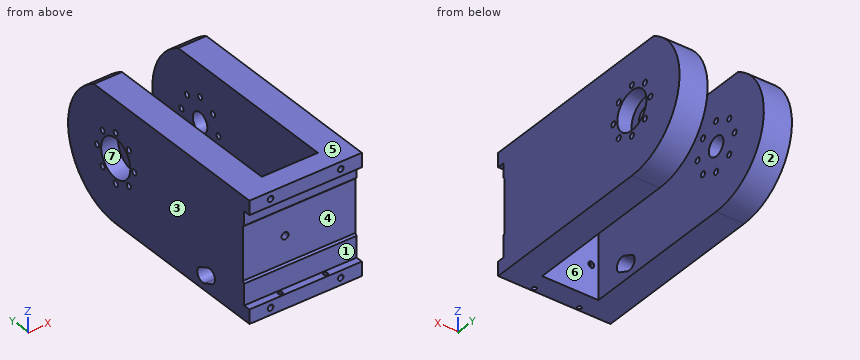
from build123d import *

# Parameters (mm, degrees)
BOSS_EXTRUDE1_DEPTH          = 101.6
CUT_EXTRUDE1_DEPTH           = 264.20443605
CUT_EXTRUDE1_DEPTH_BACK      = 264.20443605
SKETCH5_R                    = 17.4625
CUT_EXTRUDE4_DEPTH           = 15.24
CUT_EXTRUDE5_DEPTH           = 264.20443605
CUT_EXTRUDE5_DEPTH_BACK      = 264.20443605
SKETCH6_R                    = 8.73125
CUT_EXTRUDE6_START           = -12.85875
SKETCH7_R                    = 17.4625
CUT_EXTRUDE6_DEPTH           = 12.85875
F_1_4_20_TAPPED_HOLE1_D      = 5.1054
F_1_4_20_TAPPED_HOLE1_DEPTH  = 16.51
F_1_4_20_TAPPED_HOLE1_TIP    = 1.533816902
F_10_24_TAPPED_HOLE1_D       = 3.7973
F_10_24_TAPPED_HOLE1_DEPTH   = 14.9479
F_10_24_TAPPED_HOLE1_TIP     = 1.140824014
F_1_4_0_25_DIAMETER_HOLE1_D  = 6.35
F_10_0_1935_DIAMETER_HOLE1_D = 4.9149
CUT_EXTRUDE7_REACH           = 256.481
F_1_4_20_TAPPED_HOLE2_D      = 5.1054
F_1_4_20_TAPPED_HOLE2_DEPTH  = 16.51
F_1_4_20_TAPPED_HOLE2_TIP    = 1.533816902


with BuildPart() as part:
    # Sketch1 → Boss-Extrude1 (new body)
    with BuildSketch(Plane(origin=(0, 0, 0), x_dir=(0, 0, -1), z_dir=(1, 0, 0))):
        with BuildLine():
            Line((107.95, 160.3375), (107.95, 0))
            Line((107.95, 0), (95.25, 0))
            Line((95.25, 0), (95.25, 6.35))
            Line((95.25, 6.35), (76.2, 6.35))
            Line((76.2, 6.35), (74.6125, 7.9375))
            Line((74.6125, 7.9375), (26.9875, 7.9375))
            Line((26.9875, 7.9375), (25.4, 6.35))
            Line((25.4, 6.35), (12.7, 6.35))
            Line((12.7, 6.35), (12.7, 0))
            Line((12.7, 0), (0, 0))
            Line((0, 0), (0, 186.519220723))
            ThreePointArc((0, 186.519220723), (64.270384182, 215.877316798), (107.95, 160.3375))
        make_face()
    extrude(amount=BOSS_EXTRUDE1_DEPTH)

    # Sketch2 → Cut-Extrude1 (cut, two sides: drawn at the far end of the back side and taken through both)
    with BuildSketch(Plane(origin=(0, 0, -107.95), x_dir=(-1, 0, 0), z_dir=(0, 0, -1)).offset(-CUT_EXTRUDE1_DEPTH_BACK)):
        Polygon((-76.2, 98.425), (-76.2, 19.05), (-25.4, 19.05), (-25.4, 264.580157132), (-76.2, 264.580157132), align=None)
    extrude(amount=CUT_EXTRUDE1_DEPTH + CUT_EXTRUDE1_DEPTH_BACK, mode=Mode.SUBTRACT)

    # Sketch5 → Cut-Extrude4 (cut)
    with BuildSketch(Plane.ZY):
        with Locations((-50.8, 160.3375)):
            Circle(SKETCH5_R)
    extrude(amount=-CUT_EXTRUDE4_DEPTH, mode=Mode.SUBTRACT)

    # Sketch6 → Cut-Extrude5 (cut, two sides: drawn at the far end of the back side and taken through both)
    with BuildSketch(Plane.ZY.offset(-CUT_EXTRUDE5_DEPTH_BACK)):
        with Locations((-50.8, 160.3375)):
            Circle(SKETCH6_R)
    extrude(amount=CUT_EXTRUDE5_DEPTH + CUT_EXTRUDE5_DEPTH_BACK, mode=Mode.SUBTRACT)

    # Sketch7 → Cut-Extrude6 (cut)
    with BuildSketch(Plane(origin=(101.6, 0, 0), x_dir=(0, 0, -1), z_dir=(1, 0, 0)).offset(CUT_EXTRUDE6_START)):
        with Locations(Location((50.8, 160.3375, 0), (0, 0, 180))):
            Circle(SKETCH7_R)
    extrude(amount=CUT_EXTRUDE6_DEPTH, mode=Mode.SUBTRACT)

    # 1/4-20 Tapped Hole1
    with Locations(Plane(origin=(0, 0, 0), x_dir=(-1, 0, 0), z_dir=(0, -1, 0))):
        with Locations((-19.05, 6.35), (-82.55, 6.35), (-82.55, 101.6), (-19.05, 101.6)):
            Hole(F_1_4_20_TAPPED_HOLE1_D / 2, depth=F_1_4_20_TAPPED_HOLE1_DEPTH)
            with Locations((0, 0, -(F_1_4_20_TAPPED_HOLE1_DEPTH + F_1_4_20_TAPPED_HOLE1_TIP / 2))):  # 118° drill point
                Cone(0, F_1_4_20_TAPPED_HOLE1_D / 2, F_1_4_20_TAPPED_HOLE1_TIP, mode=Mode.SUBTRACT)

    # #10-24 Tapped Hole1
    with Locations(Plane(origin=(0, 0, -107.95), x_dir=(-1, 0, 0), z_dir=(0, 0, -1))):
        with Locations((-71.12, 3.175), (-30.48, 3.175)):
            Hole(F_10_24_TAPPED_HOLE1_D / 2, depth=F_10_24_TAPPED_HOLE1_DEPTH)
            with Locations((0, 0, -(F_10_24_TAPPED_HOLE1_DEPTH + F_10_24_TAPPED_HOLE1_TIP / 2))):  # 118° drill point
                Cone(0, F_10_24_TAPPED_HOLE1_D / 2, F_10_24_TAPPED_HOLE1_TIP, mode=Mode.SUBTRACT)

    # 1/4 (0.25) Diameter Hole1 (through all)
    with Locations(Plane(origin=(0, 19.05, 0), x_dir=(1, 0, 0), z_dir=(0, 1, 0))):
        with Locations((38.1, 50.8)):
            Hole(F_1_4_0_25_DIAMETER_HOLE1_D / 2)

    # #10 (0.1935) Diameter Hole1 (through all)
    with Locations(Plane.ZY):
        with Locations((-50.8, 138.1125), (-35.084551788, 144.622051788), (-28.575, 160.3375), (-35.084551788, 176.052948212), (-50.8, 182.5625), (-66.515448212, 176.052948212), (-73.025, 160.3375), (-66.515448212, 144.622051788)):
            Hole(F_10_0_1935_DIAMETER_HOLE1_D / 2)

    # Sketch18 → Cut-Extrude7 (cut, up to next)
    with BuildSketch(Plane(origin=(25.4, 0, 0), x_dir=(0, 0, -1), z_dir=(1, 0, 0)), mode=Mode.PRIVATE) as cut_extrude7_sk1:
        with BuildLine():
            Line((101.735693597, 53.742371613), (97.861527071, 45.040851129))
            ThreePointArc((97.861527071, 45.040851129), (89.477735732, 41.822615156), (86.259499759, 50.206406496))
            Line((86.259499759, 50.206406496), (90.133666285, 58.90792698))
            ThreePointArc((90.133666285, 58.90792698), (98.517457624, 62.126162953), (101.735693597, 53.742371613))
        make_face()
    cut_extrude7_tool1 = extrude(cut_extrude7_sk1.sketch, amount=-CUT_EXTRUDE7_REACH, mode=Mode.PRIVATE) & part.part
    add(cut_extrude7_tool1.solids().sort_by_distance((25.4, 51.974389, -93.997597))[0], mode=Mode.SUBTRACT)

    # 1/4-20 Tapped Hole2
    with Locations(Plane(origin=(0, 56.009710981, -24.937129984), x_dir=(1, 0, 0), z_dir=(0, 0.9135454576426035, -0.40673664307579466))):
        with Locations((31.75, 64.91550659)):
            Hole(F_1_4_20_TAPPED_HOLE2_D / 2, depth=F_1_4_20_TAPPED_HOLE2_DEPTH)
            with Locations((0, 0, -(F_1_4_20_TAPPED_HOLE2_DEPTH + F_1_4_20_TAPPED_HOLE2_TIP / 2))):  # 118° drill point
                Cone(0, F_1_4_20_TAPPED_HOLE2_D / 2, F_1_4_20_TAPPED_HOLE2_TIP, mode=Mode.SUBTRACT)


solid = part.part
Geometry check sheet. Reference: the model listing, model coordinates, mm. Face numbers are marked on the shaded views. A direction names the side the tool comes from. Coordinates: 2 decimals unless noted, no trailing zeros. Loops run counter-clockwise (first coordinate to the right, second up) from the corner with the lowest first, then second, coordinate; pieces in that order, holes last. Notation, with made-up numbers: (-32.5, 17.25) - (-20.5, 17.25) arc R24 ccw to (-20.5, 30.25) - close; hole circle Ø9 at (-39, 51.25). An arc over 180 degrees is marked (long way). Use one line per item in the form item = value. Start each with the question number.
Item 1: Section check C-C, the plane z = -50.8. Give the number of separate pieces and of enclosed holes in the cut face, and give its area (3 significant figures).
Item 2: Gauge pin test, flat ends, axial feed: pin 1 (3 mm diameter, centred on x = 63, z = -43.5, fed in from +Y); pin 2 (21 mm diameter, centred on x = 60.5, z = -84, fed in from -Y); pin 3 (8.5 mm diameter, centred on x = 38.1, z = -50.8, fed in from -Y). Record the tip position at first contact, or that the pin passes through.
Item 3: Mould release check, pull along Z, two halves, no side actions. Record for the marked faces 1, 2, 3 and 4: +Z half, -Z half, draft (parallel to the pull), parting line (faces both ways), or undercut.
Item 4: Tool access check on the marked faces 5, 6 and 7. Record the directions out of +Z, -Z, +X, -X, +Y, -Y that give a thin tool (end or side, any length) a straight path to the whole face; none if there is none.
Item 5: Thickness scan on probe 1 along Z at (x, y) = (19, 6); probe 2 along X at (y, z) = (71, -62); probe 3 along Y at (x, z) = (21, -50.8). Record the ranges inside material, lowest first.
Item 6: Section check A-A, the plane y = 133.5. Enter the section's corners in (x, z).
Item 7: Section check D-D, the plane x = 55.5. Enter the section's corners in (y, z), and give its area (3 significant figures).
Computed:
q1.separate_pieces = 8
q1.enclosed_holes = 0
q1.area = 9,260 mm2
q2.pin_1 = 19.05
q2.pin_2 = 6.35
q2.pin_3 = 7.94
q3.face_1 = undercut
q3.face_2 = parting line
q3.face_3 = draft
q3.face_4 = undercut
q4.face_5 = +Z, +X, -X, +Y, -Y
q4.face_6 = +Z, -Z, +Y
q4.face_7 = -X
q5.probe_1 = -107.95 to -104.15, -99.05 to -95.25, -12.7 to -8.9, -3.8 to 0
q5.probe_2 = 0 to 25.4, 76.2 to 101.6
q5.probe_3 = 7.94 to 135.66, 140.57 to 151.61, 169.07 to 180.11, 185.02 to 217.49
q6.outline = (0, -107.95) - (25.4, -107.95) - (25.4, 0) - (0, 0) - close; (76.2, -107.95) - (101.6, -107.95) - (101.6, 0) - (76.2, 0) - close
q7.outline = (0, -107.95) - (19.05, -107.95) - (19.05, 0) - (0, 0) - (0, -12.7) - (6.35, -12.7) - (6.35, -25.4) - (7.94, -26.99) - (7.94, -74.61) - (6.35, -76.2) - (6.35, -95.25) - (0, -95.25) - close
q7.area = 1,450 mm2
